Part model, mm, in its own coordinate system. Face numbers are marked on the shaded views. A direction names the side the tool comes from. Round coordinates to 2 decimals unless told otherwise and drop trailing zeros. Order: outer loops, then holes, each group sorted by start corner. A loop starts at its lowest first (then second) coordinate and runs counter-clockwise, first axis right, second up. Notation, with made-up numbers: (31.25, 70) - (63.25, 70) arc R15 cw to (63.25, 85) - close; hole circle Ø5 at (34.5, -35.5). An arc over 180 degrees is marked (long way). Answer as a JSON object with one key per item and string values.
```python
from build123d import *

# Parameters (mm, degrees)
SKETCH1_W               = 40
SKETCH1_H               = 20
BOSS_EXTRUDE1_DEPTH     = 10
FILLET1_R               = 3
SKETCH3_R               = 30
BOSS_EXTRUDE2_DEPTH     = 12.5
FILLET2_R               = 3
SKETCH5_R               = 2.524516272
CUT_EXTRUDE1_DEPTH      = 72.589105477
SKETCH6_W               = 7.7
SKETCH6_H               = 20
BOSS_EXTRUDE3_DEPTH     = 22
CUT_EXTRUDE3_DEPTH      = 76.359621305
CUT_EXTRUDE3_DEPTH_BACK = 76.359621305
SKETCH7_R               = 3
FILLET3_R               = 2


with BuildPart() as part:
    # Sketch1 → Boss-Extrude1 (new, symmetric)
    with BuildSketch(Plane(origin=(0, 0, 0), x_dir=(1, 0, 0), z_dir=(0, 1, 0))):
        Rectangle(SKETCH1_W, SKETCH1_H)
    extrude(amount=BOSS_EXTRUDE1_DEPTH, both=True)

    # Fillet1
    fillet1_edges = [part.edges().sort_by_distance(p)[0] for p in [
        (20, 10, 0),
        (-20, 10, 0),
        (20, -10, 0),
        (-20, -10, 0),
    ]]
    fillet(fillet1_edges, radius=FILLET1_R)

    # Sketch3 → Boss-Extrude2 (add, symmetric)
    with BuildSketch(Plane(origin=(0, 0, 0), x_dir=(1, 0, 0), z_dir=(0, 1, 0))):
        with Locations(Location((0, 30, 0), (0, 0, 270))):
            Circle(SKETCH3_R)
    extrude(amount=BOSS_EXTRUDE2_DEPTH, both=True)

    # Fillet2
    fillet2_edges = [part.edges().sort_by_distance(p)[0] for p in [
        (0, -12.5, -60),
        (0, 12.5, -60),
    ]]
    fillet(fillet2_edges, radius=FILLET2_R)

    # Sketch5 → Cut-Extrude1 (cut, through all)
    with BuildSketch(Plane(origin=(0, 12.5, 0), x_dir=(1, 0, 0), z_dir=(0, 1, 0))):
        with Locations(Location((0, 42.75, 0), (0, 0, 270))):
            Circle(SKETCH5_R)
        with Locations(Location((11.041823898, 36.375, 0), (0, 0, 270))):
            Circle(SKETCH5_R)
        with Locations(Location((11.041823898, 23.625, 0), (0, 0, 270))):
            Circle(SKETCH5_R)
        with Locations(Location((0, 17.25, 0), (0, 0, 270))):
            Circle(SKETCH5_R)
        with Locations(Location((-11.041823898, 23.625, 0), (0, 0, 270))):
            Circle(SKETCH5_R)
        with Locations(Location((-11.041823898, 36.375, 0), (0, 0, 270))):
            Circle(SKETCH5_R)
    extrude(amount=-CUT_EXTRUDE1_DEPTH, mode=Mode.SUBTRACT)

    # Sketch6 → Boss-Extrude3 (add)
    with BuildSketch(Plane.XY.offset(10)):
        with Locations((-10, 0)):
            Rectangle(SKETCH6_W, SKETCH6_H)
        with Locations((10, 0)):
            Rectangle(SKETCH6_W, SKETCH6_H)
    extrude(amount=BOSS_EXTRUDE3_DEPTH)

    # Sketch7 → Cut-Extrude3 (cut, two sides: drawn at the far end of the back side and taken through both)
    with BuildSketch(Plane.ZY.offset(13.85).offset(-CUT_EXTRUDE3_DEPTH_BACK)):
        with Locations(Location((24.5, 0, 0), (0, 0, 270))):
            Circle(SKETCH7_R)
    extrude(amount=CUT_EXTRUDE3_DEPTH + CUT_EXTRUDE3_DEPTH_BACK, mode=Mode.SUBTRACT)

    # Fillet3
    fillet3_edges = [part.edges().sort_by_distance(p)[0] for p in [
        (-10, 10, 32),
        (-10, -10, 32),
        (10, 10, 32),
        (10, -10, 32),
    ]]
    fillet(fillet3_edges, radius=FILLET3_R)


solid = part.part
```
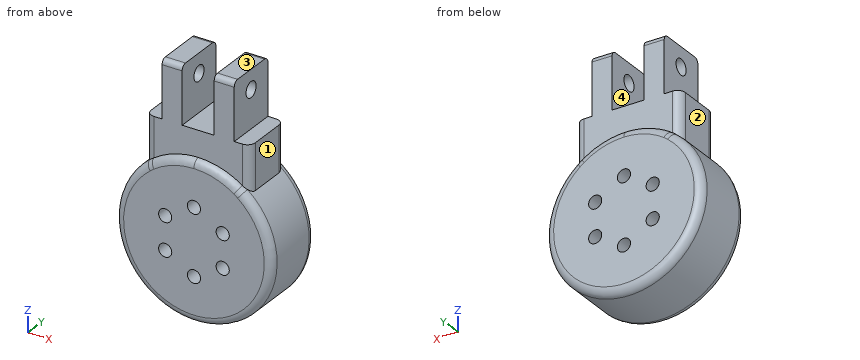
Item 1: Cut at B-B (y = -1.25). State how many separate pieces and enclosed holes the cut face has, plus the area to 3 significant figures.
Taken from the geometry:
{"separate pieces": "3", "enclosed holes": "6", "area": "3,460 mm2"}
Item 2: Cut at A-A (z = 24.5). Write the cut outline in (x, y).
Taken from the geometry:
{"outline": "(-13.85, -10) - (-6.15, -10) - (-6.15, -3) - (-13.85, -3) - close; (-13.85, 3) - (-6.15, 3) - (-6.15, 10) - (-13.85, 10) - close; (6.15, -10) - (13.85, -10) - (13.85, -3) - (6.15, -3) - close; (6.15, 3) - (13.85, 3) - (13.85, 10) - (6.15, 10) - close"}
Item 3: Drop flat-ended pins along their axis: P1, Ø1, axis at y = -3.5, z = -9, coming from the -X side; P2, Ø8, axis at y = 5, z = 10.5, coming from the -X side; P3, Ø4.5, axis at x = 11.04, z = -36.38, coming from the -Y side; P4, Ø1, axis at y = -3.5, z = -50, coming from the -X side. Give the stop position or say it passes through.
Taken from the geometry:
{"P1": "x = -21.9", "P2": "x = -20", "P3": "through", "P4": "x = -22.8"}
Item 4: Cut at C-C (y = 6). Write the cut outline in (x, z) (3 decimals).
Taken from the geometry:
{"outline": "(-20, -7.639) arc R30 ccw (long way) to (20, -7.639) - (20, 10) - (13.85, 10) - (13.85, 32) - (6.15, 32) - (6.15, 10) - (-6.15, 10) - (-6.15, 32) - (-13.85, 32) - (-13.85, 10) - (-20, 10) - close; hole circle Ø5.049 at (-11.042, -36.375); hole circle Ø5.049 at (-11.042, -23.625); hole circle Ø5.049 at (0, -42.75); hole circle Ø5.049 at (0, -17.25); hole circle Ø5.049 at (11.042, -36.375); hole circle Ø5.049 at (11.042, -23.625)"}
Item 5: Probe L1, parallel to Y at x = -11, z = 24.5; L2, parallel to X at y = -4, z = -35; L3, parallel to X at y = 8.75, z = -36.5. List the from-to ranges inside material, lowest first. Write a range as from..to.
Taken from the geometry:
{"L1": "-10..-3, 3..10", "L2": "-29.58..-13.16, -8.92..8.92, 13.16..29.58", "L3": "-29.29..-13.56, -8.52..8.52, 13.56..29.29"}
Item 6: Tool access for the marked faces 1, 2, 3 and 4: list every direction of +Z, -Z, +X, -X, +Y, -Y with a clear straight run to the whole face (end or side of a thin tool).
Taken from the geometry:
{"face 1": "+Z, +X, +Y, -Y", "face 2": "+Z, -X, +Y, -Y", "face 3": "+Z, +X, -X, +Y, -Y", "face 4": "+Z, +Y, -Y"}
